Verification items for the finished model (mm, model axes). Face numbers are marked on the shaded views. A direction names the side the tool comes from. Round coordinates to 2 decimals unless told otherwise and drop trailing zeros. Loops run counter-clockwise (first coordinate to the right, second up) from the corner with the lowest first, then second, coordinate; pieces in that order, holes last. Notation, with made-up numbers: (27, -35.75) -> (61, -35.75) arc R26 ccw to (61, -13.75) -> close; hole circle Ø5 at (73, -10.5). An arc over 180 degrees is marked (long way). Write item = value, one per line.
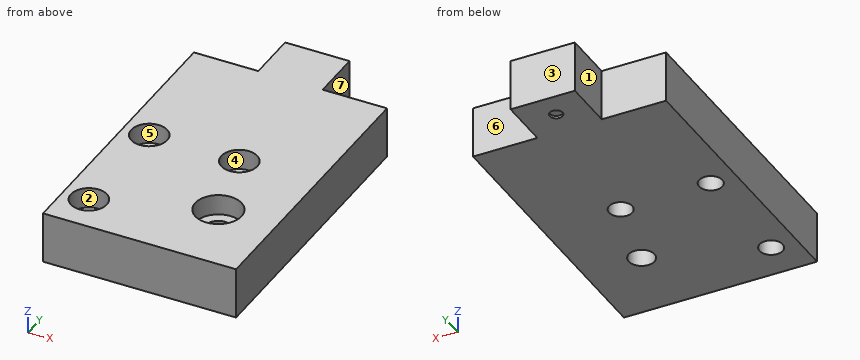
```python
from build123d import *

# Parameters (mm, degrees)
SKETCH1_R           = 2.286
SKETCH1_R_2         = 2.54
BOSS_EXTRUDE1_DEPTH = 10.16
SKETCH7_R           = 3.556
SKETCH7_R_2         = 4.572
CUT_EXTRUDE1_DEPTH  = 4.064
SKETCH3_R           = 1.27
CUT_EXTRUDE2_DEPTH  = 0.508


with BuildPart() as part:
    # Sketch1 → Boss-Extrude1 (new body)
    with BuildSketch(Plane.XY):
        Polygon((0, 57.15), (12.7, 57.15), (12.7, 67.31), (25.4, 67.31), (25.4, 57.15), (38.1, 57.15), (38.1, 0), (0, 0), align=None)
        with Locations((5.08, 7.62)):
            Circle(SKETCH1_R, mode=Mode.SUBTRACT)
        with Locations((5.08, 30.48)):
            Circle(SKETCH1_R, mode=Mode.SUBTRACT)
        with Locations((26.67, 15.24)):
            Circle(SKETCH1_R_2, mode=Mode.SUBTRACT)
        with Locations((22.86, 30.48)):
            Circle(SKETCH1_R, mode=Mode.SUBTRACT)
    extrude(amount=BOSS_EXTRUDE1_DEPTH)

    # Sketch7 → Cut-Extrude1 (cut)
    with BuildSketch(Plane.XY.offset(10.16)):
        with Locations((5.08, 30.48)):
            Circle(SKETCH7_R)
        with Locations((22.86, 30.48)):
            Circle(SKETCH7_R)
        with Locations((5.08, 7.62)):
            Circle(SKETCH7_R)
        with Locations((26.67, 15.24)):
            Circle(SKETCH7_R_2)
    extrude(amount=-CUT_EXTRUDE1_DEPTH, mode=Mode.SUBTRACT)

    # Sketch3 → Cut-Extrude2 (cut)
    with BuildSketch(Plane(origin=(0, 0, 0), x_dir=(-1, 0, 0), z_dir=(0, 0, -1))):
        with Locations((-19.05, 62.23)):
            Circle(SKETCH3_R)
    extrude(amount=-CUT_EXTRUDE2_DEPTH, mode=Mode.SUBTRACT)


solid = part.part
```
(1) Sectioned sample at D-D, the plane y = 7.62. Record the cut outline in (x, z), and give its area (3 significant figures).
Filled sheet:
outline = (0, 0) -> (2.79, 0) -> (2.79, 6.1) -> (1.52, 6.1) -> (1.52, 10.16) -> (0, 10.16) -> close; (7.37, 0) -> (38.1, 0) -> (38.1, 10.16) -> (8.64, 10.16) -> (8.64, 6.1) -> (7.37, 6.1) -> close
area = 330 mm2
(2) Material ranges on probe 1 along Y at (x, z) = (22.86, 4.75); probe 2 along Y at (x, z) = (5.08, 3); probe 3 along Y at (x, z) = (6, 5.25), recorded low to high. Write a range as from..to.
Filled sheet:
probe_1 = 0..28.19, 32.77..67.31
probe_2 = 0..5.33, 9.91..28.19, 32.77..57.15
probe_3 = 0..5.53, 9.71..28.39, 32.57..57.15
(3) Sectioned sample at C-C, the plane z = 9.5. Record the cut outline in (x, y), and give its area (3 significant figures).
Filled sheet:
outline = (0, 0) -> (38.1, 0) -> (38.1, 57.15) -> (25.4, 57.15) -> (25.4, 67.31) -> (12.7, 67.31) -> (12.7, 57.15) -> (0, 57.15) -> close; hole circle Ø7.11 at (5.08, 7.62); hole circle Ø7.11 at (5.08, 30.48); hole circle Ø7.11 at (22.86, 30.48); hole circle Ø9.14 at (26.67, 15.24)
area = 2,120 mm2
(4) Draft check along X on the marked faces 4, 5, 6 and 7. Enter one of: released by +X, released by -X, zero draft, split by the parting line, or undercut.
Filled sheet:
face_4 = undercut
face_5 = undercut
face_6 = zero draft
face_7 = released by +X
(5) Go/stop test with flat-tipped pins: pin 1 Ø3.5 at (x, y) = (24, 30) entering from +Z; pin 2 Ø5 at (x, z) = (28.5, 5) entering from +Y; pin 3 Ø5 at (y, z) = (60.5, 5.5) entering from -X. Record where each tip stops, or that it passes through.
Filled sheet:
pin_1 = 6.1
pin_2 = 57.15
pin_3 = 12.7
(6) Sectioned sample at A-A, the plane y = 30.48. Record the cut outline in (x, z), and give its area (3 significant figures).
Filled sheet:
outline = (0, 0) -> (2.79, 0) -> (2.79, 6.1) -> (1.52, 6.1) -> (1.52, 10.16) -> (0, 10.16) -> close; (7.37, 0) -> (20.57, 0) -> (20.57, 6.1) -> (19.3, 6.1) -> (19.3, 10.16) -> (8.64, 10.16) -> (8.64, 6.1) -> (7.37, 6.1) -> close; (25.15, 0) -> (38.1, 0) -> (38.1, 10.16) -> (26.42, 10.16) -> (26.42, 6.1) -> (25.15, 6.1) -> close
area = 274 mm2
(7) Sectioned sample at B-B, the plane x = 5.08. Record the cut outline in (y, z).
Filled sheet:
outline = (0, 0) -> (5.33, 0) -> (5.33, 6.1) -> (4.06, 6.1) -> (4.06, 10.16) -> (0, 10.16) -> close; (9.91, 0) -> (28.19, 0) -> (28.19, 6.1) -> (26.92, 6.1) -> (26.92, 10.16) -> (11.18, 10.16) -> (11.18, 6.1) -> (9.91, 6.1) -> close; (32.77, 0) -> (57.15, 0) -> (57.15, 10.16) -> (34.04, 10.16) -> (34.04, 6.1) -> (32.77, 6.1) -> close
(8) Set-up check for the marked faces 1, 2 and 3: record each of +Z, -Z, +X, -X, +Y, -Y from which the full face is reachable in a straight line by a thin tool's end or side.
Filled sheet:
face_1 = +Z, -Z, -X, +Y
face_2 = +Z
face_3 = +Z, -Z, +X, -X, +Y
